```python
from build123d import *

# Parameters (mm, degrees)
SKETCH_1_R      = 19.5
SKETCH_1_R_2    = 18
EXTRUDE_1_DEPTH = 10
SKETCH_3_R      = 30
EXTRUDE_2_DEPTH = 3


with BuildPart() as part:
    # 草圖1 → 填料-伸長1 (new body)
    with BuildSketch(Plane(origin=(0, 0, 0), x_dir=(1, 0, 0), z_dir=(0, 1, 0))):
        Circle(SKETCH_1_R)
        Circle(SKETCH_1_R_2, mode=Mode.SUBTRACT)
    extrude(amount=EXTRUDE_1_DEPTH)

    # 草圖3 → 填料-伸長2 (add)
    with BuildSketch(Plane.XZ):
        Circle(SKETCH_3_R)
    extrude(amount=EXTRUDE_2_DEPTH)


solid = part.part
```
For this review, take the finished solid that the model builds, in its own axes (mm). A direction names the side the tool comes from. Round coordinates to 2 decimals unless told otherwise and drop trailing zeros. Write each loop counter-clockwise with the first axis right and the second up, starting at its lowest first coordinate (ties: lowest second). Pieces come first, ordered by that corner, then holes. Notation, with made-up numbers: (39.25, -9.5) - (66.25, -9.5) arc R9 ccw to (66.25, -1.5) - close; hole circle Ø5 at (3, 74.25). An arc over 180 degrees is marked (long way). Write each question's results on one line, items separated by ' | '.
Item 1: Take a section at C-C on y = 4.5. State the section outline as (x, z) points, then the cut area to 3 significant figures.
Calculated:
outline: circle Ø39 at (0, 0); hole circle Ø36 at (0, 0) | area: 177 mm^2
Item 2: Take a section at A-A on z = 0. State the section outline as (x, y) points, then the cut area to 3 significant figures.
Calculated:
outline: (-30, -3) - (30, -3) - (30, 0) - (19.5, 0) - (19.5, 10) - (18, 10) - (18, 0) - (-18, 0) - (-18, 10) - (-19.5, 10) - (-19.5, 0) - (-30, 0) - close | area: 210 mm^2
Item 3: Take a section at D-D on x = 22. State the section outline as (y, z) points.
Calculated:
outline: (-3, -20.4) - (0, -20.4) - (0, 20.4) - (-3, 20.4) - close
Item 4: For faces 4 (the face through (5.69, 10, 17.24)), 5 (the face through (0, 0, -20)), list the 3-axis set-ups (+Z, -Z, +X, -X, +Y, -Y) from which the entire face can be reached by the end or side of a thin tool; tool diameter is ignored.
Calculated:
face 4: +Z, -Z, +X, -X, +Y | face 5: +Y
Item 5: Draft analysis for pull direction X (two halves, no side actions). For faces 1 (the face through (0, -3, 0)), 2 (the face through (0, 0, 0)), 3 (the face through (-29.97, -1.48, 1.32)), state which applies: pulls with the +X half, pulls with the -X half, needs draft (parallel to the pull), parting line crosses it, or undercut.
Calculated:
face 1: needs draft | face 2: undercut | face 3: parting line crosses it
Item 6: Take a section at B-B on x = 0. State the section outline as (y, z) points, then the cut area to 3 significant figures.
Calculated:
outline: (-3, -30) - (0, -30) - (0, -19.5) - (10, -19.5) - (10, -18) - (0, -18) - (0, 18) - (10, 18) - (10, 19.5) - (0, 19.5) - (0, 30) - (-3, 30) - close | area: 210 mm^2
Item 7: For pin 1 (8 mm diameter, centred on x = 6, z = 1.5, fed in from +Y); pin 2 (3 mm diameter, centred on y = -1, z = 18.5, fed in from +X); pin 3 (6 mm diameter, centred on y = -1, z = -20.5, fed in from +X), all flat-tipped, find the tip position at first contact; note any pin that passes through.
Calculated:
pin 1: stops at y = 0 | pin 2: stops at x = 24.72 | pin 3: stops at x = 24.37
Item 8: To check wall thickness, follow line 1 along X through (y, z) = (6, 0); line 2 along Y through (x, z) = (22.5, -11.5). State the ranges of each line that lie inside material, in increasing order. Write a range as from..to.
Calculated:
line 1: x = -19.5..-18, 18..19.5 | line 2: y = -3..0
